For this review, take the finished solid that the model builds, in its own axes (mm). A direction names the side the tool comes from. Round coordinates to 2 decimals unless told otherwise and drop trailing zeros. Write each loop counter-clockwise with the first axis right and the second up, starting at its lowest first coordinate (ties: lowest second). Pieces come first, ordered by that corner, then holes. Notation, with made-up numbers: M -18.5,80 L 14.5,80 A17 ccw 14.5,92 Z; hole C -39,-36.75 d5. An arc over 180 degrees is marked long. Use one line per item in the form item = value. Start each with the question number.
Item 1: Add section B-B (z = 27). State the section outline as (x, y) points, and give its area (3 significant figures).
Item 2: For line 1 (Z direction, x = 1.5, y = 12); line 2 (Y direction, x = -10, z = -29); line 3 (Z direction, x = -53, y = 7.5), list the stretches that pass through material, from the lowest coordinate up. Write a range as [from, to].
Item 3: For P1, Ø3, axis at y = -2.5, z = 45.5, coming from the -X side; P2, Ø1, axis at y = 0.5, z = -35.5, coming from the -X side; P3, Ø1, axis at x = 41.5, y = -2, coming from the +Z side; P4, Ø1.5, axis at x = 37, y = 0.5, coming from the -Z side, all flat-tipped, find the tip position at first contact; note any pin that passes through.
Item 4: Draft analysis for pull direction X (two halves, no side actions). For faces 3 (the conical face through (-24.426, 11.801, -0.811)), 4 (the cylindrical face through (52.482, 0.83, 52.871)), 5 (the conical face through (-1.99, 11.8, 25.18)), 6 (the conical face through (29.574, 11.801, -0.811)), state which applies: released by +X, released by -X, zero draft, split by the parting line, or undercut.
Item 5: Add section D-D (z = 0). State the section outline as (x, y) points.
Item 6: For faces 1 (the flat face through (-60, 1, 0)), 2 (the flat face through (-1, 8.225, -1)), list the 3-axis set-ups (+Z, -Z, +X, -X, +Y, -Y) from which the entire face can be reached by the end or side of a thin tool; tool diameter is ignored.
Item 7: Add section C-C (x = 0). State the section outline as (y, z) points, and give its area (3 significant figures).
Item 8: Add section A-A (x = -27). State the section outline as (y, z) points.
from build123d import *

# Parameters (mm, degrees)
CROQUIS2_W                        = 12
CROQUIS2_H                        = 12
PLATAFORMA_DEPTH                  = 1.5
REDONDEO3_R                       = 2.5
CROQUIS16_R                       = 0.4
SALIENTE_EXTRUIR7_DEPTH           = 0.5
SALIENTE_EXTRUIR7_DRAFT           = 20
SALIENTE_EXTRUIR7_PROFILE_2_DEPTH = 0.5
SALIENTE_EXTRUIR7_PROFILE_2_DRAFT = 20
SALIENTE_EXTRUIR7_PROFILE_3_DEPTH = 0.5
SALIENTE_EXTRUIR7_PROFILE_3_DRAFT = 20
SALIENTE_EXTRUIR7_PROFILE_4_DEPTH = 0.5
SALIENTE_EXTRUIR7_PROFILE_4_DRAFT = 20
ESCALA1_SCALE                     = 10


with BuildPart() as part:
    # Croquis2 → Plataforma (new body)
    with BuildSketch(Plane(origin=(0, 0, 0), x_dir=(1, 0, 0), z_dir=(0, 1, 0))):
        Rectangle(CROQUIS2_W, CROQUIS2_H)
    extrude(amount=PLATAFORMA_DEPTH)

    # Redondeo3
    redondeo3_edges = [part.edges().sort_by_distance(p)[0] for p in [
        (-6, 0.75, -6),
        (6, 0.75, -6),
        (6, 0.75, 6),
        (-6, 0.75, 6),
    ]]
    fillet(redondeo3_edges, radius=REDONDEO3_R)


with BuildPart() as saliente_extruir7_tool:
    # Croquis16 → Saliente-Extruir7 (with draft: the straight prism first)
    with BuildSketch(Plane(origin=(0, 1.5, 0), x_dir=(1, 0, 0), z_dir=(0, 1, 0))):
        with Locations((-2.7, 0)):
            Circle(CROQUIS16_R)
    extrude(amount=SALIENTE_EXTRUIR7_DEPTH)
    # Saliente-Extruir7: the draft: its side faces are tilted about the plane it starts from
    saliente_extruir7_sides = [saliente_extruir7_tool.faces().sort_by_distance(p)[0] for p in [
        (-3.1, 1.75, 0),
    ]]
    draft(saliente_extruir7_sides, Plane(origin=(0, 1.5, 0), x_dir=(1, 0, 0), z_dir=(0, 1, 0)), SALIENTE_EXTRUIR7_DRAFT)


with BuildPart() as part_1:
    add(part.part)

    # Saliente-Extruir7: add saliente_extruir7_tool
    add(saliente_extruir7_tool.part)


with BuildPart() as saliente_extruir7_profile_2_tool:
    # Croquis16 → Saliente-Extruir7 profile 2 (with draft: the straight prism first)
    with BuildSketch(Plane(origin=(0, 1.5, 0), x_dir=(1, 0, 0), z_dir=(0, 1, 0))):
        with Locations((0, -2.7)):
            Circle(CROQUIS16_R)
    extrude(amount=SALIENTE_EXTRUIR7_PROFILE_2_DEPTH)
    # Saliente-Extruir7 profile 2: the draft: its side faces are tilted about the plane it starts from
    saliente_extruir7_profile_2_sides = [saliente_extruir7_profile_2_tool.faces().sort_by_distance(p)[0] for p in [
        (-0.4, 1.75, 2.7),
    ]]
    draft(saliente_extruir7_profile_2_sides, Plane(origin=(0, 1.5, 0), x_dir=(1, 0, 0), z_dir=(0, 1, 0)), SALIENTE_EXTRUIR7_PROFILE_2_DRAFT)


with BuildPart() as part_2:
    add(part_1.part)

    # Saliente-Extruir7 profile 2: add saliente_extruir7_profile_2_tool
    add(saliente_extruir7_profile_2_tool.part)


with BuildPart() as saliente_extruir7_profile_3_tool:
    # Croquis16 → Saliente-Extruir7 profile 3 (with draft: the straight prism first)
    with BuildSketch(Plane(origin=(0, 1.5, 0), x_dir=(1, 0, 0), z_dir=(0, 1, 0))):
        with Locations((2.7, 0)):
            Circle(CROQUIS16_R)
    extrude(amount=SALIENTE_EXTRUIR7_PROFILE_3_DEPTH)
    # Saliente-Extruir7 profile 3: the draft: its side faces are tilted about the plane it starts from
    saliente_extruir7_profile_3_sides = [saliente_extruir7_profile_3_tool.faces().sort_by_distance(p)[0] for p in [
        (2.3, 1.75, 0),
    ]]
    draft(saliente_extruir7_profile_3_sides, Plane(origin=(0, 1.5, 0), x_dir=(1, 0, 0), z_dir=(0, 1, 0)), SALIENTE_EXTRUIR7_PROFILE_3_DRAFT)


with BuildPart() as part_3:
    add(part_2.part)

    # Saliente-Extruir7 profile 3: add saliente_extruir7_profile_3_tool
    add(saliente_extruir7_profile_3_tool.part)


with BuildPart() as saliente_extruir7_profile_4_tool:
    # Croquis16 → Saliente-Extruir7 profile 4 (with draft: the straight prism first)
    with BuildSketch(Plane(origin=(0, 1.5, 0), x_dir=(1, 0, 0), z_dir=(0, 1, 0))):
        with Locations((0, 2.7)):
            Circle(CROQUIS16_R)
    extrude(amount=SALIENTE_EXTRUIR7_PROFILE_4_DEPTH)
    # Saliente-Extruir7 profile 4: the draft: its side faces are tilted about the plane it starts from
    saliente_extruir7_profile_4_sides = [saliente_extruir7_profile_4_tool.faces().sort_by_distance(p)[0] for p in [
        (-0.4, 1.75, -2.7),
    ]]
    draft(saliente_extruir7_profile_4_sides, Plane(origin=(0, 1.5, 0), x_dir=(1, 0, 0), z_dir=(0, 1, 0)), SALIENTE_EXTRUIR7_PROFILE_4_DRAFT)


with BuildPart() as part_4:
    add(part_3.part)

    # Saliente-Extruir7 profile 4: add saliente_extruir7_profile_4_tool
    add(saliente_extruir7_profile_4_tool.part)


with BuildPart() as part_5:
    # Escala1: scaled about (0, 0.752818482, 0)
    add(part_4.part.scale(ESCALA1_SCALE).moved(Location((0, -6.775366338, 0))))


solid = part_5.part
Calculated:
q1.outline = M -60,-6.78 L 60,-6.78 L 60,8.22 L 4,8.22 L 2.18,13.22 L -2.18,13.22 L -4,8.22 L -60,8.22 Z
q1.area = 1,830 mm^2
q2.line_1 = [-29.16, -24.84], [24.84, 29.16]
q2.line_2 = [-6.78, 8.22]
q2.line_3 = [-52.35, 52.35]
q3.P1 = -58.32
q3.P2 = -60
q3.P3 = 59.27
q3.P4 = -59.97
q4.face_3 = undercut
q4.face_4 = released by +X
q4.face_5 = split by the parting line
q4.face_6 = undercut
q5.outline = M -60,-6.78 L 60,-6.78 L 60,8.22 L 31,8.22 L 29.18,13.22 L 24.82,13.22 L 23,8.22 L -23,8.22 L -24.82,13.22 L -29.18,13.22 L -31,8.22 L -60,8.22 Z
q6.face_1 = +Z, -Z, -X, +Y, -Y
q6.face_2 = +Y
q7.outline = M -6.78,-60 L 8.22,-60 L 8.22,-31 L 13.22,-29.18 L 13.22,-24.82 L 8.22,-23 L 8.22,23 L 13.22,24.82 L 13.22,29.18 L 8.22,31 L 8.22,60 L -6.78,60 Z
q7.area = 1,860 mm^2
q8.outline = M -6.78,-60 L 8.22,-60 L 8.22,-4 L 13.22,-2.18 L 13.22,2.18 L 8.22,4 L 8.22,60 L -6.78,60 Z
